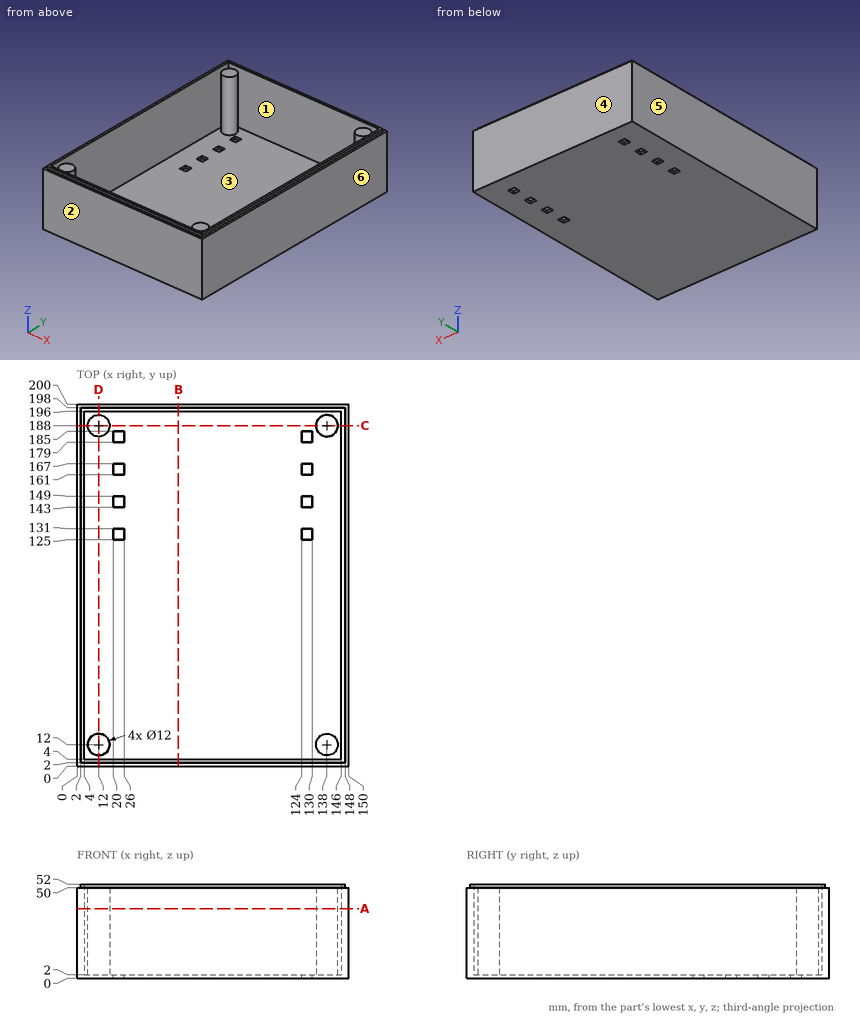
Study the drawing (mm; zero at the part's minimum x, y, z) and answer. A direction names the side the tool comes from. Give positions to 0.01 mm unless a question says otherwise; leave off trailing zeros. Write each loop counter-clockwise with the first axis right and the second up, starting at its lowest first coordinate (ties: lowest second). Pieces come first, ordered by that corner, then holes.
Item 1: Section D-D, the plane x = 12 is taken. Write down the section's boundary in (y, z), plus the area to 3 significant figures.
Item 2: Section C-C, the plane y = 188 is taken. Write down the section's boundary in (x, z).
Item 3: Find the intervals of material crossed by line 1 along X through (y, z) = (23, 48); line 2 along Y through (x, z) = (137.5, 46); line 3 along Y through (x, z) = (90.5, 34.5), in increasing order.
Item 4: Flat-ended cylindrical pins translate along their axes: P1, Ø3, axis at x = 16.5, y = 127, coming from the +Z side; P2, Ø3.5, axis at x = 9, y = 190.5, coming from the +Z side; P3, Ø2, axis at y = 51.5, z = 51.5, coming from the +X side. Find the tip coordinate at first contact, or state that the pin passes through.
Item 5: Section A-A, the plane z = 38.5 is taken. Write down the section's boundary in (x, y).
Item 6: Section B-B, the plane x = 56 is taken. Write down the section's boundary in (y, z), plus the area to 3 significant figures.
Item 7: Which of the six approach directions +Z, -Z, +X, -X, +Y, -Y give full straight-line access (tool end or side, diameter ignored) to the marked faces 1 and 2?
Item 8: Determine the mould class of the marked faces 3, 4, 5 and 6 for opening direction X: released by +X, released by -X, zero draft, split by the parting line, or undercut.
Completed:
1. outline: (0, 0) - (200, 0) - (200, 50) - (198, 50) - (198, 52) - (196, 52) - (196, 2) - (194, 2) - (194, 50) - (182, 50) - (182, 2) - (18, 2) - (18, 50) - (6, 50) - (6, 2) - (4, 2) - (4, 52) - (2, 52) - (2, 50) - (0, 50) - close
1. area: 1,940 mm2
2. outline: (0, 0) - (150, 0) - (150, 50) - (148, 50) - (148, 52) - (146, 52) - (146, 2) - (144, 2) - (144, 50) - (132, 50) - (132, 2) - (18, 2) - (18, 50) - (6, 50) - (6, 2) - (4, 2) - (4, 52) - (2, 52) - (2, 50) - (0, 50) - close
3. line 1: x = 0 to 4, 146 to 150
3. line 2: y = 0 to 4, 6.02 to 17.98, 182.02 to 193.98, 196 to 200
3. line 3: y = 0 to 4, 196 to 200
4. P1: stops at z = 2
4. P2: stops at z = 50
4. P3: stops at x = 148
5. outline: (0, 0) - (150, 0) - (150, 200) - (0, 200) - close; circle Ø12 at (12, 12); circle Ø12 at (12, 188); circle Ø12 at (138, 12); circle Ø12 at (138, 188); hole (4, 4) - (146, 4) - (146, 196) - (4, 196) - close
6. outline: (0, 0) - (200, 0) - (200, 50) - (198, 50) - (198, 52) - (196, 52) - (196, 2) - (4, 2) - (4, 52) - (2, 52) - (2, 50) - (0, 50) - close
6. area: 792 mm2
7. face 1: +Z
7. face 2: +Z, -Z, +X, -X, -Y
8. face 3: undercut
8. face 4: zero draft
8. face 5: released by -X
8. face 6: released by +X
